```python
from build123d import *

# Parameters (mm, degrees)
SKETCH1_W           = 50
SKETCH1_H           = 30
BOSS_EXTRUDE1_DEPTH = 40
CUT_EXTRUDE15_DEPTH = 40
SKETCH33_W          = 38
SKETCH33_H          = 27.886890423
CUT_EXTRUDE16_DEPTH = 1
SKETCH36_W          = 3
SKETCH36_H          = 30
CUT_EXTRUDE17_DEPTH = 40
SKETCH37_W          = 36
SKETCH37_H          = 26
BOSS_EXTRUDE5_DEPTH = 1
SKETCH38_W          = 6
SKETCH38_H          = 3
BOSS_EXTRUDE6_DEPTH = 1


with BuildPart() as part:
    # Sketch1 → Boss-Extrude1 (new body)
    with BuildSketch(Plane.XY):
        with Locations((-9.745762712, 0.593220339)):
            Rectangle(SKETCH1_W, SKETCH1_H)
    extrude(amount=BOSS_EXTRUDE1_DEPTH)

    # Sketch29 → Cut-Extrude15 (cut)
    with BuildSketch(Plane.XY.offset(40)):
        Polygon((-34.745762712, -11.406779661), (-19.745762712, 15.593220339), (-34.745762712, 15.593220339), align=None)
    extrude(amount=-CUT_EXTRUDE15_DEPTH, mode=Mode.SUBTRACT)

    # Sketch33 → Cut-Extrude16 (cut)
    with BuildSketch(Plane(origin=(-21.708506556, 12.06028142, 0), x_dir=(0, 0, 1), z_dir=(-0.874157276, 0.485642931, 0))):
        with Locations((20, -11.401908276)):
            Rectangle(SKETCH33_W, SKETCH33_H)
    extrude(amount=-CUT_EXTRUDE16_DEPTH, mode=Mode.SUBTRACT)

    # Sketch36 → Cut-Extrude17 (cut)
    with BuildSketch(Plane.XY.offset(40)):
        with Locations((13.754237288, 0.593220339)):
            Rectangle(SKETCH36_W, SKETCH36_H)
    extrude(amount=-CUT_EXTRUDE17_DEPTH, mode=Mode.SUBTRACT)

    # Sketch37 → Boss-Extrude5 (add)
    with BuildSketch(Plane(origin=(12.254237288, 0, 0), x_dir=(0, 0, -1), z_dir=(1, 0, 0))):
        with Locations((-20, 0.593220339)):
            Rectangle(SKETCH37_W, SKETCH37_H)
    extrude(amount=BOSS_EXTRUDE5_DEPTH)

    # Sketch38 → Boss-Extrude6 (add)
    with BuildSketch(Plane(origin=(13.254237288, 0, 0), x_dir=(0, 0, -1), z_dir=(1, 0, 0))):
        with Locations((-20, -12.906779661)):
            Rectangle(SKETCH38_W, SKETCH38_H)
    extrude(amount=BOSS_EXTRUDE6_DEPTH)


solid = part.part
```
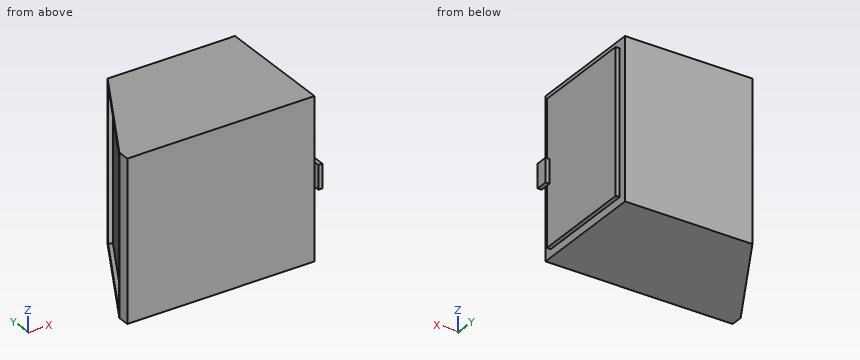
Can you work these out from the model? Positions are in its coordinate system, mm. Give positions to 0.01 mm unless a question says otherwise; leave off trailing zeros. Order: outer loops, then holes, each group sorted by start corner. A loop starts at its lowest first (then second) coordinate and runs counter-clockwise, first axis right, second up. Notation, with made-up numbers: M 20,53.25 L 46,53.25 A27 cw 46,79.25 Z; hole C 50,-4 d7. An arc over 180 degrees is marked long. Write item = value, one per line. Start each with the question number.
Q1. Will these pins go through, and if not, where does the flat tip stop? pin 1 Ø0.8 at (x, y) = (14, -13.5) entering from +Z; pin 2 Ø12 at (y, z) = (4.5, 30.5) entering from -X; pin 3 Ø1 at (x, z) = (-20.5, 27) entering from +Y.
Q2. I need wall thicknesses on probe 1 along X at (y, z) = (10.5, 27); probe 2 along X at (y, z) = (10, 31); probe 3 along Y at (x, z) = (-28.5, 9.5). Which ranges of each line are inside material? Lowest first, please. Write a range as [from, to].
Q3. Suppose I cut it at C-C (x = -29). Write out the boundary of the cut face in (y, z), plus the area to 3 significant figures.
Q4. Suppose I cut it at A-A (z = 27). Write out the boundary of the cut face in (x, y).
Q5. Suppose I cut it at D-D (z = 19). Write out the boundary of the cut face in (x, y).
Q6. Suppose I cut it at B-B (y = -6). Write out the boundary of the cut face in (x, z), plus the area to 3 significant figures.
Check result:
q1.pin_1 = 23
q1.pin_2 = -28.1
q1.pin_3 = 15.14
q2.probe_1 = [-21.43, 13.25]
q2.probe_2 = [-21.71, 13.25]
q2.probe_3 = [-14.41, -2.22]
q3.outline = M -14.41,0 L -1.06,0 L -1.06,1 L -3.12,1 L -3.12,39 L -1.06,39 L -1.06,40 L -14.41,40 Z
q3.area = 455 mm2
q4.outline = M -34.75,-14.41 L 12.25,-14.41 L 12.25,-12.41 L 13.25,-12.41 L 13.25,13.59 L 12.25,13.59 L 12.25,15.59 L -19.75,15.59 L -20.47,14.28 L -19.6,13.8 L -33.14,-10.58 L -34.02,-10.1 L -34.75,-11.41 Z
q5.outline = M -34.75,-14.41 L 12.25,-14.41 L 12.25,-12.41 L 13.25,-12.41 L 13.25,-14.41 L 14.25,-14.41 L 14.25,-11.41 L 13.25,-11.41 L 13.25,13.59 L 12.25,13.59 L 12.25,15.59 L -19.75,15.59 L -20.47,14.28 L -19.6,13.8 L -33.14,-10.58 L -34.02,-10.1 L -34.75,-11.41 Z
q6.outline = M -31.74,0 L 12.25,0 L 12.25,2 L 13.25,2 L 13.25,38 L 12.25,38 L 12.25,40 L -31.74,40 L -31.74,39 L -30.6,39 L -30.6,1 L -31.74,1 Z
q6.area = 1,750 mm2
